Geometry: see drawing. Coordinates: mm, zero at the bounding-box minimum. A direction names the side the tool comes from. Give positions to 0.01 mm unless a question says otherwise; leave off trailing zeros. Write each loop counter-clockwise with the first axis right and the second up, starting at its lowest first coordinate (ties: lowest second). Pieces come first, ordered by that corner, then holes. Notation, with made-up numbers: M 76.25,-24 L 83.25,-24 A19 ccw 83.25,-18 Z; hole C 75,-11.5 d4. An arc over 180 degrees is marked long. Use a Markdown table: item, result. Add a question column.
1) Section D-D on y = 19. Return the cut outline in (x, z), then the cut area to 3 significant figures.
2) Set-up query: the marked faces 4 and 5. Return all of +Z, -Z, +X, -X, +Y, -Y with unobstructed straight access to the full face (end or side cutting, diameter ignored); none if empty.
3) Section B-B on z = 10. Return the cut outline in (x, y).
4) Section A-A on y = 96. Return the cut outline in (x, z).
5) Line query: line 1 (Z direction, x = 14.5, y = 134.5) (1 decimal); line 2 (Z direction, x = 36, y = 146); line 3 (Z direction, x = 29, y = 146.5) (1 decimal). Output: solid intervals per line, ascending.
6) Draft query along Z for the marked faces 1, 2 and 3. Return one class per face: +Z half, -Z half, draft (parallel to the pull), parting line (faces both ways), or undercut.
7) Pin query (flat end, axial travel): pin 1 (2.5 mm diameter, centred on y = 7, z = 35.5, fed in from +X); pin 2 (2 mm diameter, centred on y = 26.5, z = 23, fed in from +X); pin 3 (1.5 mm diameter, centred on y = 19.5, z = 35.5, fed in from -X). Return the tip coordinate at first contact, or that it passes through.
8) Section C-C on x = 38. Return the cut outline in (y, z), then the cut area to 3 significant figures.
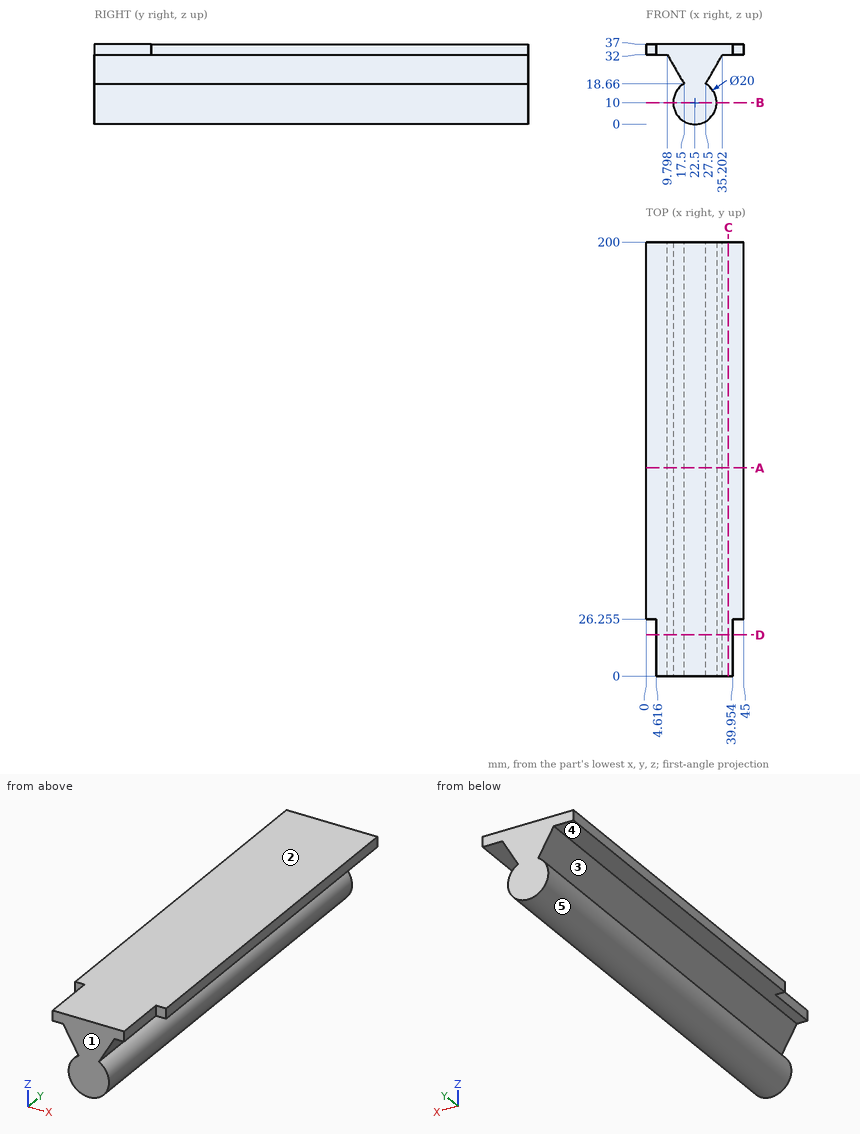
Found:
| question | item | result |
|---|---|---|
| 1 | outline | M 4.62,32 L 9.8,32 L 17.5,18.66 A10 ccw long 27.5,18.66 L 35.2,32 L 39.95,32 L 39.95,37 L 4.62,37 Z |
| 1 | area | 718 mm² |
| 2 | face 4 | -Z, -X, +Y, -Y |
| 2 | face 5 | +Y, -Y |
| 3 | outline | M 12.5,0 L 32.5,0 L 32.5,200 L 12.5,200 Z |
| 4 | outline | M 0,32 L 9.8,32 L 17.5,18.66 A10 ccw long 27.5,18.66 L 35.2,32 L 45,32 L 45,37 L 0,37 Z |
| 5 | line 1 | 4 to 16, 23.9 to 37 |
| 5 | line 2 | 32 to 37 |
| 5 | line 3 | 2.4 to 17.6, 21.3 to 37 |
| 6 | face 1 | draft |
| 6 | face 2 | +Z half |
| 6 | face 3 | undercut |
| 7 | pin 1 | x = 39.95 |
| 7 | pin 2 | x = 30.58 |
| 7 | pin 3 | x = 4.62 |
| 8 | outline | M 0,32 L 200,32 L 200,37 L 0,37 Z |
| 8 | area | 1,000 mm² |
